Print and shaded views of the part. All mm, measured from the part's lowest x, y and z. A direction names the side the tool comes from. Round coordinates to 2 decimals unless told otherwise and drop trailing zeros. Loops run counter-clockwise (first coordinate to the right, second up) from the corner with the lowest first, then second, coordinate; pieces in that order, holes last. Notation, with made-up numbers: (13.25, 67) -> (33.25, 67) arc R9 cw to (33.25, 77) -> close; hole circle Ø4 at (0, 28.5). An arc over 180 degrees is marked (long way). Use a Markdown table: item, result.
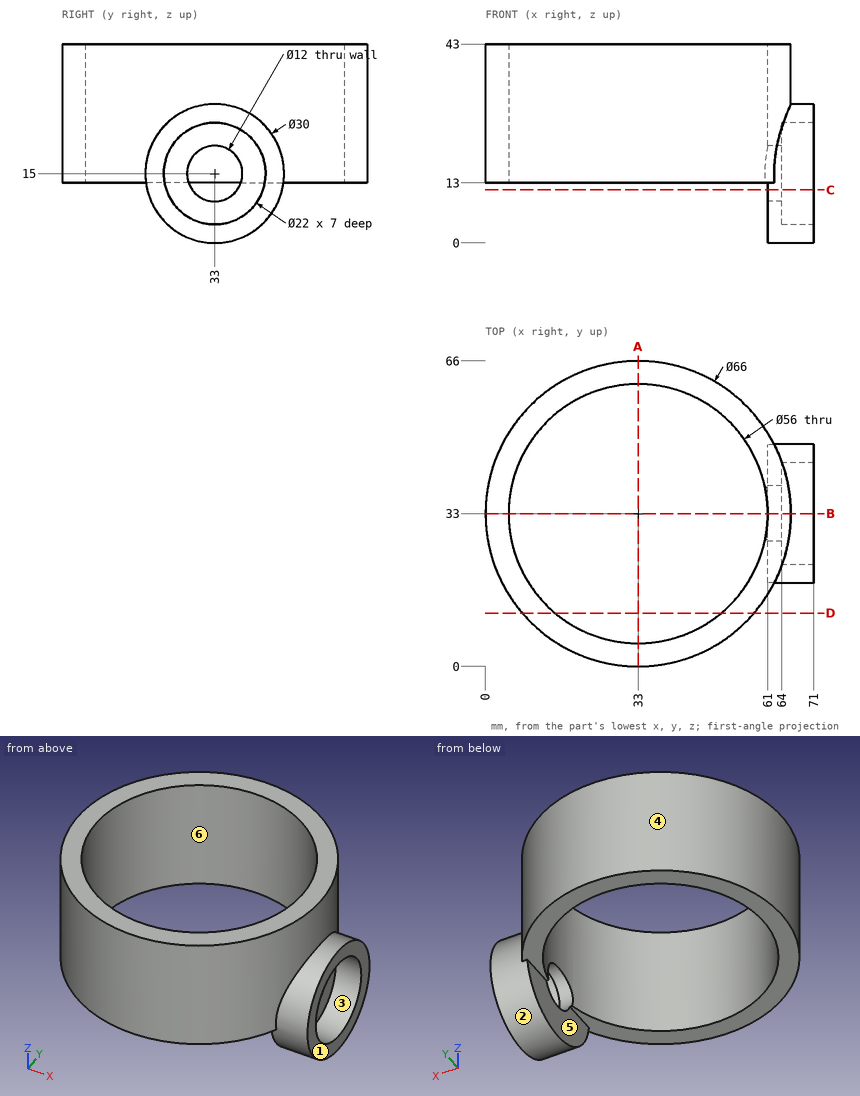
Q1. Band-saw the part on B-B, the plane y = 33. Give the cut face in (x, z).
Results list:
| item | result |
|---|---|
| outline | (0, 13) -> (5, 13) -> (5, 43) -> (0, 43) -> close; (61, 0) -> (71, 0) -> (71, 4) -> (64, 4) -> (64, 9) -> (61, 9) -> close; (61, 21) -> (64, 21) -> (64, 26) -> (71, 26) -> (71, 30) -> (66, 30) -> (66, 43) -> (61, 43) -> close |
Q2. Tool access for the marked faces 1 and 2: list every direction of +Z, -Z, +X, -X, +Y, -Y with a clear straight run to the whole face (end or side of a thin tool).
Results list:
| item | result |
|---|---|
| face 1 | +Z, -Z, +X, +Y, -Y |
| face 2 | +X |
Q3. Flat gauge pins, fed straight in: pin 1 (6 mm diameter, centred on x = 53, z = 14.5, fed in from -Y); pin 2 (10.5 mm diameter, centred on y = 32, z = 4.5, fed in from -X); pin 3 (5 mm diameter, centred on y = 14.5, z = 13, fed in from -X); pin 4 (24 mm diameter, centred on y = 32.5, z = 13.5, fed in from +X). Where does each tip first touch, or does it go through?
Results list:
| item | result |
|---|---|
| pin 1 | stops at y = 4.72 |
| pin 2 | stops at x = 61 |
| pin 3 | stops at x = 4.14 |
| pin 4 | stops at x = 71 |
Q4. Drill centre lines: L1, parallel to Y at x = 66.5, z = 15; L2, parallel to Y at x = 32, z = 28; L3, parallel to X at y = 39, z = 33. Where is each one in solid material? Low to high. Write a range as from..to.
Results list:
| item | result |
|---|---|
| L1 | y = 18..22, 44..48 |
| L2 | y = 0.02..5.02, 60.98..65.98 |
| L3 | x = 0.55..5.65, 60.35..65.45 |
Q5. Band-saw the part on D-D, the plane y = 11.5. Give the cut face in (x, z).
Results list:
| item | result |
|---|---|
| outline | (7.97, 13) -> (15.06, 13) -> (15.06, 43) -> (7.97, 43) -> close; (50.94, 13) -> (58.03, 13) -> (58.03, 43) -> (50.94, 43) -> close |
Q6. Band-saw the part on A-A, the plane x = 33. Give the cut face in (y, z), plus the area to 3 significant figures.
Results list:
| item | result |
|---|---|
| outline | (0, 13) -> (5, 13) -> (5, 43) -> (0, 43) -> close; (61, 13) -> (66, 13) -> (66, 43) -> (61, 43) -> close |
| area | 300 mm² |
Q7. Pull direction X, two halves, no side cores. Call the marked faces 3, 4, 5 and 6: released by +X, released by -X, zero draft, split by the parting line, or undercut.
Results list:
| item | result |
|---|---|
| face 3 | zero draft |
| face 4 | split by the parting line |
| face 5 | released by -X |
| face 6 | undercut |
Q8. Band-saw the part on C-C, the plane z = 11.5. Give the cut face in (x, y).
Results list:
| item | result |
|---|---|
| outline | (61, 18.41) -> (71, 18.41) -> (71, 22.57) -> (64, 22.57) -> (64, 28.13) -> (61, 28.13) -> close; (61, 37.87) -> (64, 37.87) -> (64, 43.43) -> (71, 43.43) -> (71, 47.59) -> (61, 47.59) -> close |
